from build123d import *

# Parameters (mm, degrees)
SKETCH_1_W          = 42
SKETCH_1_H          = 42
EXTRUDE_1_DEPTH     = 40
SKETCH_2_R          = 11
EXTRUDE_2_DEPTH     = 2
SKETCH_3_R          = 2.5
EXTRUDE_5_DEPTH     = 22
SKETCH_4_R          = 1.5
CUT_EXTRUDE_1_DEPTH = 31.5
CHAMFER_2_SIZE      = 5


with BuildPart() as part:
    # ｽｹｯﾁ1 → ﾎﾞｽ - 押し出し1 (new body)
    with BuildSketch(Plane.XY):
        Rectangle(SKETCH_1_W, SKETCH_1_H)
    extrude(amount=EXTRUDE_1_DEPTH)

    # ｽｹｯﾁ2 → ﾎﾞｽ - 押し出し2 (add)
    with BuildSketch(Plane.XY.offset(40)):
        Circle(SKETCH_2_R)
    extrude(amount=EXTRUDE_2_DEPTH)

    # ｽｹｯﾁ3 → ﾎﾞｽ - 押し出し5 (add)
    with BuildSketch(Plane.XY.offset(42)):
        Circle(SKETCH_3_R)
    extrude(amount=EXTRUDE_5_DEPTH)

    # ｽｹｯﾁ4 → ｶｯﾄ - 押し出し1 (cut)
    with BuildSketch(Plane.XY.offset(40)):
        with Locations((-15.5, 15.5)):
            Circle(SKETCH_4_R)
        with Locations((15.5, 15.5)):
            Circle(SKETCH_4_R)
        with Locations((15.5, -15.5)):
            Circle(SKETCH_4_R)
        with Locations((-15.5, -15.5)):
            Circle(SKETCH_4_R)
    extrude(amount=-CUT_EXTRUDE_1_DEPTH, mode=Mode.SUBTRACT)

    # 面取り2
    chamfer_2_edges = [part.edges().sort_by_distance(p)[0] for p in [
        (21, -21, 20),
        (-21, -21, 20),
        (-21, 21, 20),
        (21, 21, 20),
    ]]
    chamfer(chamfer_2_edges, length=CHAMFER_2_SIZE)


solid = part.part
For this review, take the finished solid that the model builds, in its own axes (mm). A direction names the side the tool comes from. Coordinates: 2 decimals unless noted, no trailing zeros. Loops run counter-clockwise (first coordinate to the right, second up) from the corner with the lowest first, then second, coordinate; pieces in that order, holes last. Notation, with made-up numbers: (57.5, 46) - (74.5, 46) arc R21 ccw to (74.5, 65) - close; hole circle Ø8 at (28.25, 82). An arc over 180 degrees is marked (long way). Return JSON: item names as keys, results as strings.
Item 1: For line 1 (Y direction, x = -15.5, z = 21.5); line 2 (X direction, y = -15, z = 26); line 3 (Z direction, x = 18, y = 17.5), list the stretches that pass through material, from the lowest coordinate up.
Determined:
{"line 1": "y = -21 to -17, -14 to 14, 17 to 21", "line 2": "x = -21 to -16.91, -14.09 to 14.09, 16.91 to 21", "line 3": "z = 0 to 40"}
Item 2: Take a section at B-B (y = 0). Give the boundary of the cut face in (x, z).
Determined:
{"outline": "(-21, 0) - (21, 0) - (21, 40) - (11, 40) - (11, 42) - (2.5, 42) - (2.5, 64) - (-2.5, 64) - (-2.5, 42) - (-11, 42) - (-11, 40) - (-21, 40) - close"}
Item 3: Take a section at A-A (z = 18). Give the boundary of the cut face in (x, y).
Determined:
{"outline": "(-21, -16) - (-16, -21) - (16, -21) - (21, -16) - (21, 16) - (16, 21) - (-16, 21) - (-21, 16) - close; hole circle Ø3 at (-15.5, -15.5); hole circle Ø3 at (-15.5, 15.5); hole circle Ø3 at (15.5, -15.5); hole circle Ø3 at (15.5, 15.5)"}
Item 4: Mouldability with a two-part tool opening along X and no side actions: class faces 3 (the flat face through (-18, -19, 20)), 4 (the flat face through (0, 21, 20)), 5 (the flat face through (-16, 16, 8.5)) as pulls with the +X half, pulls with the -X half, needs draft (parallel to the pull), parting line crosses it, or undercut.
Determined:
{"face 3": "pulls with the -X half", "face 4": "needs draft", "face 5": "undercut"}
Item 5: Insertion check: pin 1 (5 mm diameter, centred on y = -1, z = 49.5, fed in from +X); pin 2 (0.9 mm diameter, centred on x = -16, y = -15, fed in from +Z); pin 3 (3.5 mm diameter, centred on x = 15, y = -16, fed in from +Z); pin 4 (2 mm diameter, centred on y = 6, z = 43.5, fed in from +X). Each pin has a flat end and moves straight along its axis. Give the tip position at first contact, or say it passes through.
Determined:
{"pin 1": "stops at x = 2.5", "pin 2": "stops at z = 8.5", "pin 3": "stops at z = 40", "pin 4": "passes through"}
Item 6: For faces 1 (the flat face through (0, 0, 64)), 2 (the cylindrical face through (-17, 15.57, 24.47)), list the 3-axis set-ups (+Z, -Z, +X, -X, +Y, -Y) from which the entire face can be reached by the end or side of a thin tool; tool diameter is ignored.
Determined:
{"face 1": "+Z, +X, -X, +Y, -Y", "face 2": "+Z"}
Item 7: Take a section at D-D (z = 57). Give the boundary of the cut face in (x, y), then the cut area to 3 significant figures.
Determined:
{"outline": "circle Ø5 at (0, 0)", "area": "19.6 mm2"}
